Geometry check sheet. Reference: the model listing, model coordinates, mm. A direction names the side the tool comes from. Round coordinates to 2 decimals unless told otherwise and drop trailing zeros. Write each loop counter-clockwise with the first axis right and the second up, starting at its lowest first coordinate (ties: lowest second). Pieces come first, ordered by that corner, then holes.
from build123d import *

# Parameters (mm, degrees)
SKETCH1_R               = 4.025
SKETCH1_R_2             = 2.125
BOSS_EXTRUDE1_DEPTH     = 2.5
SKETCH2_R               = 59
CUT_EXTRUDE1_DEPTH      = 3.5
CUT_EXTRUDE1_DEPTH_BACK = 3.5


with BuildPart() as part:
    # Sketch1 → Boss-Extrude1 (new body, symmetric)
    with BuildSketch(Plane(origin=(0, 0, 0), x_dir=(1, 0, 0), z_dir=(0, 1, 0))):
        Polygon((-55.5, 30), (-55.5, -30), (-70.5, -30), (-70.5, 30), (-36.615368979, 62.892866181), (-29.338096583, 55.396174082), align=None)
        with Locations((-37.999438908, 54.268822934)):
            Circle(SKETCH1_R, mode=Mode.SUBTRACT)
        with Locations((-63, 0)):
            Circle(SKETCH1_R_2, mode=Mode.SUBTRACT)
        with Locations((-63, -15)):
            Circle(SKETCH1_R_2, mode=Mode.SUBTRACT)
        with Locations((-63, 15)):
            Circle(SKETCH1_R_2, mode=Mode.SUBTRACT)
    extrude(amount=BOSS_EXTRUDE1_DEPTH, both=True)

    # Sketch2 → Cut-Extrude1 (cut, two sides)
    with BuildSketch(Plane(origin=(0, 0, 0), x_dir=(1, 0, 0), z_dir=(0, 1, 0))) as cut_extrude1_sk:
        Circle(SKETCH2_R)
    extrude(amount=CUT_EXTRUDE1_DEPTH, mode=Mode.SUBTRACT)
    extrude(cut_extrude1_sk.sketch, amount=-CUT_EXTRUDE1_DEPTH_BACK, mode=Mode.SUBTRACT)


solid = part.part
1. Depth check by flat-ended pin: pin 1 Ø1.5 at (y, z) = (0.5, -25.5) entering from +X; pin 2 Ø2.5 at (x, z) = (-63, 0) entering from +Y. Enter the tip coordinate at first touch or a pass-through.
2. Section check A-A (z = 15). Record the cut outline in (x, y) (3 decimals), plus the area to 3 significant figures.
3. Section check C-C (y = 0). Record the cut outline in (x, z) (3 decimals), plus the area to 3 significant figures.
4. Release check for a two-part mould opening along Z. For faces 3 (the face through (-53.79, 0.04, -46.22)), 4 (the face through (-55.5, 0, 25)), 5 (the face through (-59, 0, 0)) record: +Z half, -Z half, draft (parallel to the pull), parting line (faces both ways), or undercut.
5. Scan lines: line 1 along X through (y, z) = (1.05, 0) (3 decimals); line 2 along Z through (x, y) = (-63, -1.95) (3 decimals); line 3 along X through (y, z) = (-1.6, 23.5). Record each from-to range of solid material in increasing order.
6. Access from +Z, -Z, +X, -X, +Y, -Y to the whole of each face (thin tool, end or side, straight path). Record for faces 1 (the face through (-55.5, 0, -25)), 2 (the face through (-59, 2.5, -13)).
7. Section check D-D (z = 0). Record the cut outline in (x, y) (3 decimals), plus the area to 4 significant figures.
8. Section check B-B (x = -63). Record the cut outline in (y, z) (3 decimals), plus the area to 3 significant figures.
Results below:
1. pin 1: stops at x = -55.5
1. pin 2: passes through
2. outline: (-70.5, -2.5) - (-65.125, -2.5) - (-65.125, 2.5) - (-70.5, 2.5) - close; (-60.875, -2.5) - (-57.061, -2.5) - (-57.061, 2.5) - (-60.875, 2.5) - close
2. area: 45.9 mm2
3. outline: (-70.5, -30) - (-36.615, -62.893) - (-29.338, -55.396) - (-55.5, -30) - (-55.5, -20.019) arc R59 cw to (-55.5, 20.019) - (-55.5, 30) - (-70.5, 30) - close; hole circle Ø4.25 at (-63, -15); hole circle Ø4.25 at (-63, 0); hole circle Ø4.25 at (-63, 15); hole circle Ø8.05 at (-37.999, -54.269)
3. area: 1,150 mm2
4. face 3: -Z half
4. face 4: draft
4. face 5: undercut
5. line 1: x = -70.5 to -65.125, -60.875 to -59
5. line 2: z = -37.28 to -17.125, -12.875 to -2.125, 2.125 to 12.875, 17.125 to 30
5. line 3: x = -70.5 to -55.5
6. face 1: +Z, +X, +Y, -Y
6. face 2: +Z, -Z, +X, -X, +Y
7. outline: (-70.5, -2.5) - (-65.125, -2.5) - (-65.125, 2.5) - (-70.5, 2.5) - close; (-60.875, -2.5) - (-59, -2.5) - (-59, 2.5) - (-60.875, 2.5) - close
7. area: 36.25 mm2
8. outline: (-2.5, -37.28) - (2.5, -37.28) - (2.5, -17.125) - (-2.5, -17.125) - close; (-2.5, -12.875) - (2.5, -12.875) - (2.5, -2.125) - (-2.5, -2.125) - close; (-2.5, 2.125) - (2.5, 2.125) - (2.5, 12.875) - (-2.5, 12.875) - close; (-2.5, 17.125) - (2.5, 17.125) - (2.5, 30) - (-2.5, 30) - close
8. area: 273 mm2
